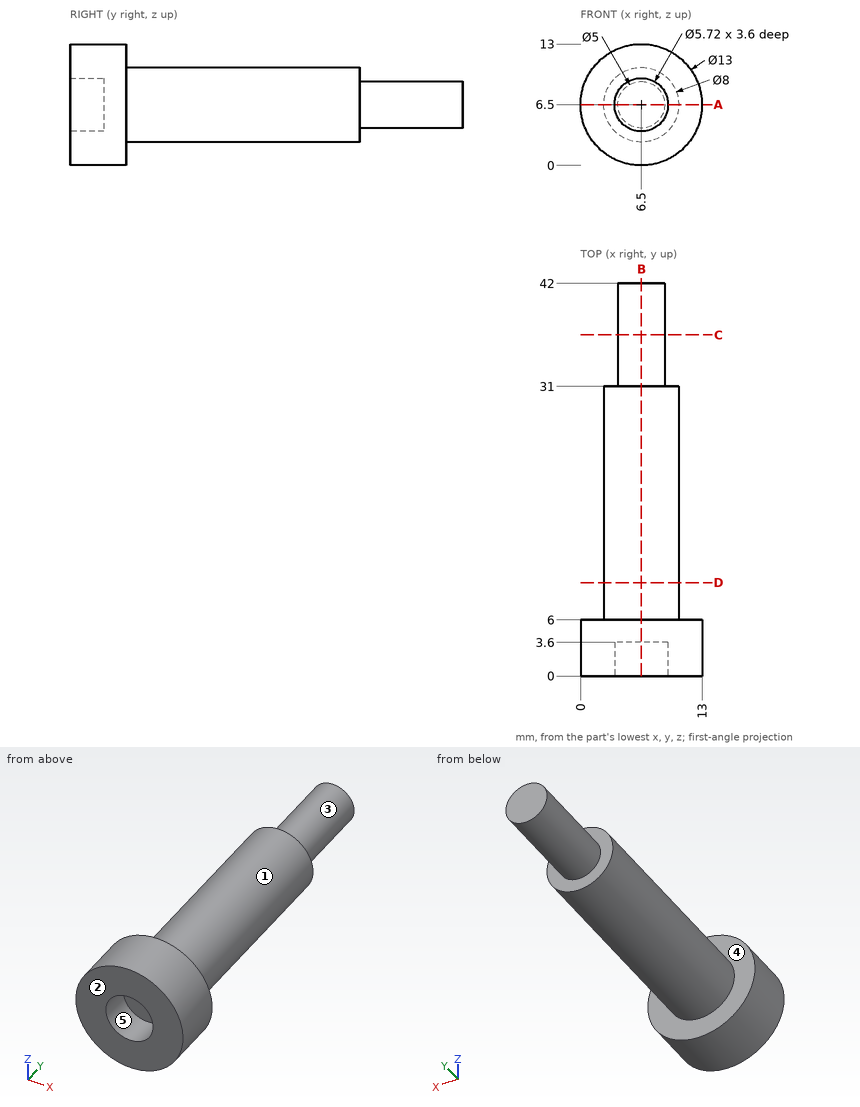
Job drawing, mm, ordinate dimensions from the low corner. One solid piece. A direction names the side the tool comes from. Round coordinates to 2 decimals unless told otherwise and drop trailing zeros. Write each loop counter-clockwise with the first axis right and the second up, starting at its lowest first coordinate (ties: lowest second). Pieces come first, ordered by that corner, then holes. Notation, with made-up numbers: M 21,11.25 L 54,11.25 A28 cw 54,49.25 Z; hole C 16.25,53.25 d5. An arc over 180 degrees is marked long. Return JSON: item names as keys, results as strings. Group by question number.
(1) Pin check, flat tips, straight feed: pin 1 Ø2 at (x, z) = (1.5, 11.5) entering from +Y; pin 2 Ø1.5 at (x, y) = (9, 30) entering from +Z; pin 3 Ø1.5 at (y, z) = (35, 2.5) entering from -X; pin 4 Ø5 at (x, z) = (11.5, 8.5) entering from +Y. Stop position of each tip, or through.
(2) Saw through at A-A on z = 6.5. Write the cut outline in (x, y), then the cut area to 3 significant figures.
(3) Saw through at B-B on x = 6.5. Write the cut outline in (y, z).
(4) Saw through at C-C on y = 36.5. Write the cut outline in (x, z), then the cut area to 3 significant figures.
(5) Drill centre lines: probe 1 along X at (y, z) = (2.35, 6.5); probe 2 along Y at (x, z) = (9.5, 10.25); probe 3 along Y at (x, z) = (7, 8.5). Where is each one in solid material? Low to high.
(6) Two-plate mould, pull along Z, no slides. Class the marked faces 3, 4 and 5: +Z half, -Z half, draft (parallel to the pull), parting line (faces both ways), or undercut.
(7) Saw through at D-D on y = 10. Write the cut outline in (x, z), then the cut area to 3 significant figures.
(8) Which spindle directions (+Z, -Z, +X, -X, +Y, -Y) get a long thin tool onto all of the face, cutting with end or side? Do the marked faces 1 and 2. Say none if no direction does.
Returned:
{
 "1": {"pin 1": "y = 6", "pin 2": "z = 10.1", "pin 3": "through", "pin 4": "y = 31"},
 "2": {"outline": "M 0,0 L 3.64,0 L 3.64,3.6 L 9.36,3.6 L 9.36,0 L 13,0 L 13,6 L 10.5,6 L 10.5,31 L 9,31 L 9,42 L 4,42 L 4,31 L 2.5,31 L 2.5,6 L 0,6 Z", "area": "312 mm²"},
 "3": {"outline": "M 0,0 L 6,0 L 6,2.5 L 31,2.5 L 31,4 L 42,4 L 42,9 L 31,9 L 31,10.5 L 6,10.5 L 6,13 L 0,13 L 0,9.36 L 3.6,9.36 L 3.6,3.64 L 0,3.64 Z"},
 "4": {"outline": "C 6.5,6.5 d5", "area": "19.6 mm²"},
 "5": {"probe 1": "0 to 3.64, 9.36 to 13", "probe 2": "0 to 6", "probe 3": "3.6 to 42"},
 "6": {"face 3": "parting line", "face 4": "draft", "face 5": "undercut"},
 "7": {"outline": "C 6.5,6.5 d8", "area": "50.3 mm²"},
 "8": {"face 1": "+Y", "face 2": "+Z, -Z, +X, -X, -Y"}
}
